```python
from build123d import *

# Parameters (mm, degrees)
SKETCH1_R           = 27.5
SKETCH1_R_2         = 3
SKETCH1_R_3         = 5
BOSS_EXTRUDE1_DEPTH = 6
FILLET1_R           = 5


with BuildPart() as part:
    # Sketch1 → Boss-Extrude1 (new body)
    with BuildSketch(Plane(origin=(0, 0, 0), x_dir=(1, 0, 0), z_dir=(0, 1, 0))):
        with BuildLine():
            Line((-123.5, 87.6), (123.5, 87.6))
            Line((123.5, 87.6), (123.5, 47.6))
            Line((123.5, 47.6), (94.604107801, 47.6))
            ThreePointArc((94.604107801, 47.6), (84.895928348, 45.085744243), (77.628633504, 38.175125172))
            Line((77.628633504, 38.175125172), (46.48038696, -11.824874828))
            ThreePointArc((46.48038696, -11.824874828), (44.426515721, -16.245001343), (43.502792816, -21.030671774))
            Line((43.502792816, -21.030671774), (39.782384757, -75.242332057))
            ThreePointArc((39.782384757, -75.242332057), (38.206473118, -78.554562921), (34.794117647, -79.9))
            Line((34.794117647, -79.9), (33.462740879, -79.9))
            ThreePointArc((33.462740879, -79.9), (29.927206973, -78.435533906), (28.462740879, -74.9))
            Line((28.462740879, -74.9), (28.462740879, -68.462740879))
            ThreePointArc((28.462740879, -68.462740879), (20.126197087, -48.336543792), (0, -40))
            ThreePointArc((0, -40), (-28.284271247, -28.284271247), (-40, 0))
            Line((-40, 0), (-40, 4.1))
            ThreePointArc((-40, 4.1), (-52.740855018, 34.859144982), (-83.5, 47.6))
            Line((-83.5, 47.6), (-123.5, 47.6))
            Line((-123.5, 47.6), (-123.5, 87.6))
        make_face()
        with Locations(Location((0, 0, 0), (0, 0, 270))):
            Circle(SKETCH1_R, mode=Mode.SUBTRACT)
        with Locations(Location((38.5, -20.9, 0), (0, 0, 270))):
            Circle(SKETCH1_R_2, mode=Mode.SUBTRACT)
        with Locations(Location((35, -71.9, 0), (0, 0, 270))):
            Circle(SKETCH1_R_2, mode=Mode.SUBTRACT)
        with Locations(Location((-103.5, 67.6, 0), (0, 0, 270))):
            Circle(SKETCH1_R_3, mode=Mode.SUBTRACT)
        with Locations(Location((103.5, 67.6, 0), (0, 0, 90))):
            Circle(SKETCH1_R_3, mode=Mode.SUBTRACT)
    extrude(amount=BOSS_EXTRUDE1_DEPTH)

    # Fillet1
    fillet1_edges = [part.edges().sort_by_distance(p)[0] for p in [
        (-123.5, 3, -87.6),
        (123.5, 3, -87.6),
        (123.5, 3, -47.6),
        (-123.5, 3, -47.6),
    ]]
    fillet(fillet1_edges, radius=FILLET1_R)


solid = part.part
```
Input: part model. Units: mm. Frame: model coordinates. A direction names the side the tool comes from. Give positions to 0.01 mm unless a question says otherwise; leave off trailing zeros. Order: outer loops, then holes, each group sorted by start corner. A loop starts at its lowest first (then second) coordinate and runs counter-clockwise, first axis right, second up. Notation, with made-up numbers: (79.5, 87) - (113.5, 87) arc R5 ccw to (113.5, 93) - close; hole circle Ø8 at (-4.5, -7.5). An arc over 180 degrees is marked (long way). One line per item, written item: value.
1. Cut plane B-B, the plane z = 4. Output: boundary loops of the cut face in (x, y) (1 decimal).
Determined:
outline: (-39.8, 0) - (-27.2, 0) - (-27.2, 6) - (-39.8, 6) - close; (27.2, 0) - (51.4, 0) - (51.4, 6) - (27.2, 6) - close
2. Line query: probe 1 along X at (y, z) = (4, -67.6); probe 2 along X at (y, z) = (3.9, 18.5); probe 3 along Z at (x, y) = (103.5, 2.45). Output: solid intervals per line, ascending.
Determined:
probe 1: -123.5 to -108.5, -98.5 to 98.5, 108.5 to 123.5
probe 2: -35.46 to -20.35, 20.35 to 36.7, 40.3 to 43.84
probe 3: -87.6 to -72.6, -62.6 to -47.6
3. Cut plane C-C, the plane x = -48.5. Output: boundary loops of the cut face in (y, z), and give its area (3 significant figures).
Determined:
outline: (0, -87.6) - (6, -87.6) - (6, -29.93) - (0, -29.93) - close
area: 346 mm2
4. Pin query (flat end, axial travel): pin 1 Ø3 at (y, z) = (3.5, 50) entering from -X; pin 2 Ø6 at (x, z) = (-103.5, -67.6) entering from -Y; pin 3 Ø1.5 at (y, z) = (1, -2) entering from -X. Return the tip coordinate at first contact, or that it passes through.
Determined:
pin 1: x = 20.29
pin 2: through
pin 3: x = -40
5. Draft query along Z for faces 1 (the face through (123.5, 3, -68)), 2 (the face through (85.02, 2.958, -45.154)), 3 (the face through (37.03, 2.96, 69.69)). Return one class per face: released by +Z, released by -Z, zero draft, split by the parting line, or undercut.
Determined:
face 1: zero draft
face 2: released by +Z
face 3: undercut
6. Cut plane A-A, the plane y = 1.1. Output: boundary loops of the cut face in (x, z), and give its area (3 significant figures).
Determined:
outline: (-123.5, -82.6) arc R5 ccw to (-118.5, -87.6) - (118.5, -87.6) arc R5 ccw to (123.5, -82.6) - (123.5, -52.6) arc R5 ccw to (118.5, -47.6) - (94.6, -47.6) arc R20 cw to (77.63, -38.18) - (46.48, 11.82) arc R20 cw to (43.5, 21.03) - (39.78, 75.24) arc R5 ccw to (34.79, 79.9) - (33.46, 79.9) arc R5 ccw to (28.46, 74.9) - (28.46, 68.46) arc R28.46 cw to (0, 40) arc R40 ccw to (-40, 0) - (-40, -4.1) arc R43.5 cw to (-83.5, -47.6) - (-118.5, -47.6) arc R5 ccw to (-123.5, -52.6) - close; hole circle Ø10 at (-103.5, -67.6); hole circle Ø55 at (0, 0); hole circle Ø6 at (35, 71.9); hole circle Ø6 at (38.5, 20.9); hole circle Ø10 at (103.5, -67.6)
area: 16,600 mm2
7. Reachability of faces 4 (the face through (107, 3, -47.6)), 5 (the face through (-101, 3, -47.6)), 6 (the face through (122, 3.04, -86.17)) from +Z, -Z, +X, -X, +Y, -Y: full face, straight path, thin tool, end or side. Return the list, or none.
Determined:
face 4: +Z, +X, +Y, -Y
face 5: +Z, -X, +Y, -Y
face 6: -Z, +X, +Y, -Y
8. Cut plane D-D, the plane z = -33.5. Output: boundary loops of the cut face in (x, y), and give its area (3 significant figures).
Determined:
outline: (-51.44, 0) - (74.72, 0) - (74.72, 6) - (-51.44, 6) - close
area: 757 mm2
